Part model, mm, in its own coordinate system. A direction names the side the tool comes from. Give positions to 0.01 mm unless a question says otherwise; leave off trailing zeros. Write each loop counter-clockwise with the first axis right and the second up, starting at its lowest first coordinate (ties: lowest second). Pieces come first, ordered by that corner, then holes. Notation, with made-up numbers: (-6, 32) - (52, 32) arc R22 cw to (52, 48) - close; hole circle Ø6 at (40, 61.5). An arc over 180 degrees is marked (long way). Answer as a JSON object with one key per item and string values. Group by question number.
```python
from build123d import *

# Parameters (mm, degrees)
BOSS_EXTRUDE1_DEPTH = 5
SKETCH2_W           = 80
SKETCH2_H           = 15
BOSS_EXTRUDE2_DEPTH = 5
SKETCH3_W           = 15
SKETCH3_H           = 15
BOSS_EXTRUDE3_DEPTH = 3
SKETCH4_W           = 15
SKETCH4_H           = 15
BOSS_EXTRUDE4_DEPTH = 3
SKETCH5_W           = 0.08
SKETCH5_H           = 10
CUT_EXTRUDE1_DEPTH  = 10
SKETCH6_W           = 10.40455395
SKETCH6_H           = 5
BOSS_EXTRUDE5_DEPTH = 5


with BuildPart() as part:
    # Sketch1 → Boss-Extrude1 (new body)
    with BuildSketch(Plane.XY):
        Polygon((-40, 10), (40, 10), (40, 0), (5, 0), (5, -65), (-5, -65), (-5, 0), (-40, 0), align=None)
    extrude(amount=BOSS_EXTRUDE1_DEPTH)

    # Sketch2 → Boss-Extrude2 (add)
    with BuildSketch(Plane(origin=(0, 10, 0), x_dir=(1, 0, 0), z_dir=(0, 1, 0))):
        with Locations((0, 2.5)):
            Rectangle(SKETCH2_W, SKETCH2_H)
    extrude(amount=BOSS_EXTRUDE2_DEPTH)

    # Sketch3 → Boss-Extrude3 (add)
    with BuildSketch(Plane(origin=(40, 0, 0), x_dir=(0, 0, -1), z_dir=(1, 0, 0))):
        with Locations((2.5, 7.5)):
            Rectangle(SKETCH3_W, SKETCH3_H)
    extrude(amount=BOSS_EXTRUDE3_DEPTH)

    # Sketch4 → Boss-Extrude4 (add)
    with BuildSketch(Plane.ZY.offset(40)):
        with Locations((-2.5, 7.5)):
            Rectangle(SKETCH4_W, SKETCH4_H)
    extrude(amount=BOSS_EXTRUDE4_DEPTH)

    # Sketch5 → Cut-Extrude1 (cut)
    with BuildSketch(Plane.XZ):
        with Locations((-40.04, -5)):
            Rectangle(SKETCH5_W, SKETCH5_H)
        with Locations((40.04, -5)):
            Rectangle(SKETCH5_W, SKETCH5_H)
    extrude(amount=-CUT_EXTRUDE1_DEPTH, mode=Mode.SUBTRACT)

    # Sketch6 → Boss-Extrude5 (add)
    with BuildSketch(Plane(origin=(0, 15, 0), x_dir=(1, 0, 0), z_dir=(0, 1, 0))):
        with Locations((-0.202276975, -2.5)):
            Rectangle(SKETCH6_W, SKETCH6_H)
    extrude(amount=BOSS_EXTRUDE5_DEPTH)


solid = part.part
```
1) Probe line 1 (X direction, y = 3, z = -4); line 2 (X direction, y = -54, z = 3.25); line 3 (Y direction, x = -3, z = -5.5). List the from-to ranges inside material, lowest first.
2) Band-saw the part on A-A (z = -2.5). List the corners of the cut face in (x, y), plus the area to 3 significant figures.
3) Band-saw the part on C-C (y = -47). List the corners of the cut face in (x, z).
4) Drop flat-ended pins along their axis: P1, Ø4, axis at y = -40, z = 2, coming from the -X side; P2, Ø4, axis at y = 18.5, z = 2, coming from the +X side; P3, Ø5, axis at x = -20, z = -7.5, coming from the +Y side; P4, Ø2, axis at y = -37.5, z = -2.5, coming from the -X side. Give the stop position or say it passes through.
5) Band-saw the part on D-D (x = 35.5). List the corners of the cut face in (y, z).
6) Mould opens along X. For faces 1 (the flat face through (-5, -33, 2)), 2 (the flat face through (0, -8, 0)), 3 (the flat face through (1, 15, -3)), 4 (the flat face through (40.08, 5, -5)) say: pulls with the +X half, pulls with the -X half, needs draft (parallel to the pull), parting line crosses it, or undercut.
7) Which spindle directions (+Z, -Z, +X, -X, +Y, -Y) get a long thin tool onto all of the face, cutting with end or side? Do faces 5 (the flat face through (0, 17, 0)), 6 (the flat face through (5, 17, 3)), 7 (the flat face through (-40.08, 5, -5)), 8 (the flat face through (5, -32, 2)). Say none if no direction does.
8) Band-saw the part on B-B (x = 3.5). List the corners of the cut face in (y, z).
Verdict:
{
 "1": {"line 1": "-43 to -40.08, 40.08 to 43", "line 2": "-5 to 5", "line 3": "10 to 15"},
 "2": {"outline": "(-43, 0) - (-40.08, 0) - (-40.08, 10) - (40.08, 10) - (40.08, 0) - (43, 0) - (43, 15) - (-43, 15) - close", "area": "488 mm2"},
 "3": {"outline": "(-5, 0) - (5, 0) - (5, 5) - (-5, 5) - close"},
 "4": {"P1": "x = -5", "P2": "x = 5", "P3": "y = 15", "P4": "through"},
 "5": {"outline": "(0, 0) - (10, 0) - (10, -10) - (15, -10) - (15, 5) - (0, 5) - close"},
 "6": {"face 1": "pulls with the -X half", "face 2": "undercut", "face 3": "needs draft", "face 4": "undercut"},
 "7": {"face 5": "-Z, +X, -X, +Y", "face 6": "+Z, -Z, +X, +Y", "face 7": "-Z, -Y", "face 8": "+Z, -Z, +X, -Y"},
 "8": {"outline": "(-65, 0) - (10, 0) - (10, -10) - (15, -10) - (15, 0) - (20, 0) - (20, 5) - (-65, 5) - close"}
}
